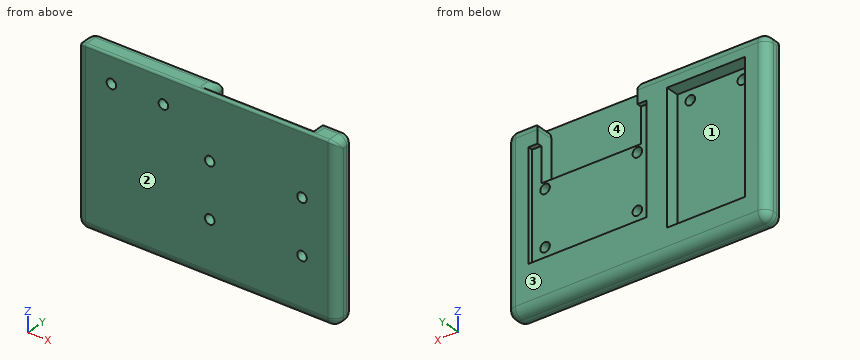
from build123d import *

# Parameters (mm, degrees)
SKETCH1_W               = 60
SKETCH1_H               = 40
BOSS_EXTRUDE1_DEPTH     = 5
SKETCH2_W               = 18
SKETCH2_H               = 30
SKETCH2_R               = 1.1
SKETCH2_W_2             = 27.3
SKETCH2_H_2             = 25
CUT_EXTRUDE1_DEPTH      = 1.1
SKETCH3_W               = 18
SKETCH3_H               = 30
SKETCH3_R               = 1.1
CUT_EXTRUDE2_DEPTH      = 2
SKETCH4_W               = 23
SKETCH4_H               = 13
CUT_EXTRUDE3_DEPTH      = 4
CUT_EXTRUDE3_DEPTH_BACK = 3
SKETCH5_R               = 1.1
CUT_EXTRUDE4_DEPTH      = 6
FILLET1_R               = 2
FILLET2_R               = 0.5


with BuildPart() as part:
    # Sketch1 → Boss-Extrude1 (new body)
    with BuildSketch(Plane(origin=(0, 0, 0), x_dir=(1, 0, 0), z_dir=(0, 1, 0))):
        Rectangle(SKETCH1_W, SKETCH1_H)
    extrude(amount=BOSS_EXTRUDE1_DEPTH)

    # Sketch2 → Cut-Extrude1 (cut)
    with BuildSketch(Plane(origin=(0, 5, 0), x_dir=(1, 0, 0), z_dir=(0, 1, 0))):
        with Locations((-16, -1.01)):
            Rectangle(SKETCH2_W, SKETCH2_H)
        with Locations((-22, -13.71)):
            Circle(SKETCH2_R, mode=Mode.SUBTRACT)
        with Locations((-10, -13.71)):
            Circle(SKETCH2_R, mode=Mode.SUBTRACT)
        with Locations((11.35, -2.5)):
            Rectangle(SKETCH2_W_2, SKETCH2_H_2)
        with Locations((0.7, 7)):
            Circle(SKETCH2_R, mode=Mode.SUBTRACT)
        with Locations((0.7, -5.5)):
            Circle(SKETCH2_R, mode=Mode.SUBTRACT)
        with Locations((22, -5.5)):
            Circle(SKETCH2_R, mode=Mode.SUBTRACT)
        with Locations((22, 7)):
            Circle(SKETCH2_R, mode=Mode.SUBTRACT)
    extrude(amount=-CUT_EXTRUDE1_DEPTH, mode=Mode.SUBTRACT)

    # Sketch3 → Cut-Extrude2 (cut)
    with BuildSketch(Plane(origin=(0, 3.9, 0), x_dir=(1, 0, 0), z_dir=(0, 1, 0))):
        with Locations((-16, -1.01)):
            Rectangle(SKETCH3_W, SKETCH3_H)
        with Locations((-10, -13.71)):
            Circle(SKETCH3_R, mode=Mode.SUBTRACT)
        with Locations((-22, -13.71)):
            Circle(SKETCH3_R, mode=Mode.SUBTRACT)
    extrude(amount=-CUT_EXTRUDE2_DEPTH, mode=Mode.SUBTRACT)

    # Sketch4 → Cut-Extrude3 (cut, two sides)
    with BuildSketch(Plane(origin=(0, 3.9, 0), x_dir=(1, 0, 0), z_dir=(0, 1, 0))) as cut_extrude3_sk:
        with Locations((11.35, -13.5)):
            Rectangle(SKETCH4_W, SKETCH4_H)
    extrude(amount=CUT_EXTRUDE3_DEPTH, mode=Mode.SUBTRACT)
    extrude(cut_extrude3_sk.sketch, amount=-CUT_EXTRUDE3_DEPTH_BACK, mode=Mode.SUBTRACT)

    # Sketch5 → Cut-Extrude4 (cut, through all)
    with BuildSketch(Plane(origin=(0, 5, 0), x_dir=(1, 0, 0), z_dir=(0, 1, 0))):
        with Locations((22, 7)):
            Circle(SKETCH5_R)
        with Locations((22, -5.5)):
            Circle(SKETCH5_R)
        with Locations((0.7, -5.5)):
            Circle(SKETCH5_R)
        with Locations((0.7, 7)):
            Circle(SKETCH5_R)
        with Locations((-10, -13.71)):
            Circle(SKETCH5_R)
        with Locations((-22, -13.71)):
            Circle(SKETCH5_R)
    extrude(amount=-CUT_EXTRUDE4_DEPTH, mode=Mode.SUBTRACT)

    # Fillet1
    fillet1_edges = [part.edges().sort_by_distance(p)[0] for p in [
        (-30, 5, 0),
        (-15.075, 5, 20),
        (30, 5, 0),
        (-30, 0, 0),
        (0, 0, -20),
        (30, 0, 0),
        (30, 2.5, 20),
        (-30, 2.5, 20),
        (-30, 2.5, -20),
        (30, 2.5, -20),
        (26.425, 5, 20),
        (-0.15, 2.95, 20),
        (22.85, 2.95, 20),
        (0, 5, -20),
    ]]
    fillet(fillet1_edges, radius=FILLET1_R)

    # Fillet2
    fillet2_edges = [part.edges().sort_by_distance(p)[0] for p in [
        (0, 0, 20),
        (29.526592034, 0.707902185, 19.292097815),
        (-29.526592034, 0.707902185, 19.292097815),
    ]]
    fillet(fillet2_edges, radius=FILLET2_R)


solid = part.part
Read the model definition and answer for the solid it produces. Units are mm, in the model's axes. Face numbers are marked on the shaded views. A direction names the side the tool comes from. Coordinates: 2 decimals unless noted, no trailing zeros. Write each loop counter-clockwise with the first axis right and the second up, starting at its lowest first coordinate (ties: lowest second). Pieces come first, ordered by that corner, then holes. Notation, with made-up numbers: (-18.5, 32.5) -> (18.5, 32.5) arc R30 ccw to (18.5, 59.5) -> close; hole circle Ø8 at (2, 44). An arc over 180 degrees is marked (long way). Return JSON: item names as keys, results as strings.
(1) For a pull along X with two mould halves and no side action, classify the marked faces 3 and 4 as pulls with the +X half, pulls with the -X half, needs draft (parallel to the pull), parting line crosses it, or undercut.
Answers below:
{"face 3": "needs draft", "face 4": "undercut"}
(2) The part is cut by section A-A on z = 5.5. Give the vertices of the cut face in (x, y), then the cut area to 3 significant figures.
Answers below:
{"outline": "(-30, 2) arc R2 ccw to (-28, 0) -> (-0.4, 0) -> (-0.4, 3.9) -> (-2.3, 3.9) -> (-2.3, 5) -> (-7, 5) -> (-7, 1.9) -> (-25, 1.9) -> (-25, 5) -> (-28, 5) arc R2 ccw to (-30, 3) -> close; (1.8, 0) -> (20.9, 0) -> (20.9, 3.9) -> (1.8, 3.9) -> close; (23.1, 0) -> (28, 0) arc R2 ccw to (30, 2) -> (30, 3) arc R2 ccw to (28, 5) -> (25, 5) -> (25, 3.9) -> (23.1, 3.9) -> close", "area": "194 mm^2"}
(3) Each of these flat-tipped pins is pushed along its axis until it touches: P1, Ø0.9, axis at x = 6, y = 2, coming from the +Z side; P2, Ø0.6, axis at x = 17, y = 4.5, coming from the +Z side; P3, Ø7.5, axis at x = 8, z = 5.5, coming from the +Y side. Where does it stop, or does it pass through?
Answers below:
{"P1": "z = 7", "P2": "z = -10", "P3": "y = 3.9"}
(4) The part is cut by section D-D on z = -1. Give the vertices of the cut face in (x, y).
Answers below:
{"outline": "(-30, 2) arc R2 ccw to (-28, 0) -> (28, 0) arc R2 ccw to (30, 2) -> (30, 3) arc R2 ccw to (28, 5) -> (25, 5) -> (25, 3.9) -> (-2.3, 3.9) -> (-2.3, 5) -> (-7, 5) -> (-7, 1.9) -> (-25, 1.9) -> (-25, 5) -> (-28, 5) arc R2 ccw to (-30, 3) -> close"}
(5) The part is cut by section B-B on x = -22. Give the vertices of the cut face in (y, z), then the cut area to 3 significant figures.
Answers below:
{"outline": "(0, -18) arc R2 ccw to (2, -20) -> (3, -20) arc R2 ccw to (5, -18) -> (5, -13.99) -> (1.9, -13.99) -> (1.9, 12.61) -> (0, 12.61) -> close; (0, 14.81) -> (1.9, 14.81) -> (1.9, 16.01) -> (5, 16.01) -> (5, 18) arc R2 ccw to (3, 20) -> (0.5, 20) arc R0.5 ccw to (0, 19.5) -> close", "area": "100 mm^2"}
(6) The part is cut by section C-C on x = 0.7. Give the vertices of the cut face in (y, z).
Answers below:
{"outline": "(0, -18) arc R2 ccw to (2, -20) -> (3, -20) arc R2 ccw to (5, -18) -> (5, -10) -> (3.9, -10) -> (3.9, -8.1) -> (0, -8.1) -> close; (0, -5.9) -> (3.9, -5.9) -> (3.9, 4.4) -> (0, 4.4) -> close; (0, 6.6) -> (3.9, 6.6) -> (3.9, 7) -> (0.9, 7) -> (0.9, 20) -> (0.5, 20) arc R0.5 ccw to (0, 19.5) -> close"}
(7) Which of the six approach directions +Z, -Z, +X, -X, +Y, -Y give full straight-line access (tool end or side, diameter ignored) to the marked faces 1 and 2?
Answers below:
{"face 1": "+Y", "face 2": "+Z, -Z, +X, -X, -Y"}
(8) Consider line 1 along Z through (x, y) = (22, 2.6); line 2 along X through (y, z) = (2.3, -12); line 3 along X through (y, z) = (3.55, 14). Determine where each line is inside the solid, lowest interval first. Write a range as from..to.
Answers below:
{"line 1": "-20..-8.1, -5.9..4.4, 6.6..7", "line 2": "-30..-25, -7..30", "line 3": "-29.92..-25, -7..-0.15, 22.85..29.92"}
